Part model, mm, in its own coordinate system. A direction names the side the tool comes from. Give positions to 0.01 mm unless a question says otherwise; leave off trailing zeros. Order: outer loops, then holes, each group sorted by start corner. A loop starts at its lowest first (then second) coordinate and runs counter-clockwise, first axis right, second up. Notation, with made-up numbers: (-7.5, 2) -> (24.5, 2) arc R30 ccw to (24.5, 32) -> close; hole circle Ø1 at (6, 70.25). An arc over 180 degrees is marked (long way). Write item = value, one per line. Start each with the question number.
(1) Saw through at D-D, the plane z = -106. List the corners of the cut face in (x, y), then the cut area to 3 significant figures.
(2) Saw through at A-A, the plane x = -41. State how many separate pieces and enclosed holes the cut face has, then the cut area to 3 significant figures.
(3) Saw through at B-B, the plane y = 33.27. List the corners of the cut face in (x, z), then the cut area to 3 significant figures.
(4) Probe line 1 along Y through (x, z) = (-23.5, -36); line 2 along Z through (x, y) = (-30, 34); line 3 along Y through (x, z) = (-6, -244.5). List the from-to ranges inside material, lowest first. Write a range as from..to.
(5) Flat gauge pins, fed straight in: pin 1 (16 mm diameter, centred on y = -4, z = -25, fed in from -X); pin 2 (1.5 mm diameter, centred on x = 36, z = 215.5, fed in from -Y); pin 3 (8 mm diameter, centred on x = -26.5, y = -24, fed in from +Z). Where does each tip first touch, or does it go through?
(6) Saw through at C-C, the plane z = 37.5. List the corners of the cut face in (x, y).
(7) Two-plate mould, pull along Z, no slides. Class faces 3 (the cylindrical face through (0.833, 31.879, 338.384)), 4 (the cylindrical face through (0.833, -14.175, -62.474)), 5 (the flat face through (-59.5, 7.6, 362.8)): pulls with the +Z half, pulls with the -Z half, needs draft (parallel to the pull), parting line crosses it, or undercut.
(8) Which spindle directions (+Z, -Z, +X, -X, +Y, -Y) get a long thin tool onto all of the face, cutting with end or side? Do faces 1 (the flat face through (-59.5, -39, 97)), 2 (the flat face through (59.5, -13, 174)). Say none if no direction does.
Autodesk Inventor part; units mm, degrees
ref_plane "YZ Plane" through (0, 0, 0) normal (1, 0, 0) x (0, 1, 0)
ref_plane "XZ Plane" through (0, 0, 0) normal (0, 1, 0) x (-1, 0, 0)
ref_plane "XY Plane" through (0, 0, 0) normal (0, 0, 1) x (1, 0, 0)
sketch "Sketch1" plane through (0, 0, 0) normal (1, 0, 0) x (0, 1, 0)
  line L0 (66.79, 404) -> (66.79, -404)
  line L1 (66.79, -404) -> (12.72, -404)
  line L2 (12.72, -404) -> (-46.497, -331.3)
  line L3 (-46.497, -331.3) -> (-46.497, 331.3)
  line L4 (-46.497, 331.3) -> (12.72, 404)
  line L5 (12.72, 404) -> (66.79, 404)
  point P0 (0, 0)
  dimension "d0" = 331.3
  dimension "d1" = 331.3
  dimension "d2" = 46.497
  dimension "d3" = 46.497
  dimension "d4" = 12.72
  dimension "d5" = 12.72
  dimension "d6" = 404
  dimension "d7" = 404
  dimension "d8" = 66.79
extrude "Extrusion1" add sketch "Sketch1" along normal blind 66.5
sketch "Sketch2" plane through (0, 0, 0) normal (-1, 0, 0) x (0, 0, 1)
  line L0 (404, 66.79) -> (-404, 66.79)
  line L1 (-404, 66.79) -> (-404, 12.72)
  line L2 (-404, 12.72) -> (-331.3, -46.497)
  line L3 (331.3, -46.497) -> (404, 12.72)
  line L4 (404, 12.72) -> (404, 66.79)
  line L5 (404, 66.79) -> (-404, 66.79)
  line L6 (-404, 66.79) -> (-404, 12.72)
  line L7 (-404, 12.72) -> (-331.3, -46.497)
  line L8 (-331.3, -46.497) -> (331.3, -46.497)
  point P0 (0, 0)
extrude "Extrusion2" cut sketch "Sketch2" against normal blind 59.5
sketch "Sketch3" plane through (59.5, 0, 0) normal (-1, 0, 0) x (0, 0, 1)
  circle A0 centre (-370.6, 33.27) radius 31.6465
  circle A1 centre (-316, -13.01) radius 31.6465
  circle A2 centre (-246, -13.01) radius 31.6465
  circle A3 centre (-176, -13.01) radius 31.6465
  circle A4 centre (-106, -13.01) radius 31.6465
  circle A5 centre (-36, -13.01) radius 31.6465
  circle A6 centre (34, -13.01) radius 31.6465
  circle A7 centre (104, -13.01) radius 31.6465
  circle A8 centre (174, -13.01) radius 31.6465
  circle A9 centre (244, -13.01) radius 31.6465
  circle A10 centre (314, -13.01) radius 31.6465
  circle A11 centre (370, 33.27) radius 31.6465
  point P0 (0, 0)
  dimension "d13" = 33.27
  dimension "d14" = 33.27
  dimension "d15" = 370.6
  dimension "d16" = 370
  dimension "d17" = 316
  dimension "d18" = 13.01
  dimension "d19" = 70
  dimension "d20" = 70
  dimension "d21" = 70
  dimension "d22" = 70
  dimension "d23" = 70
  dimension "d24" = 70
  dimension "d25" = 70
  dimension "d26" = 70
  dimension "d27" = 70
  dimension "d28" = 13.01
  dimension "d29" = 13.01
  dimension "d30" = 13.01
  dimension "d31" = 13.01
  dimension "d32" = 13.01
  dimension "d33" = 13.01
  dimension "d34" = 13.01
  dimension "d35" = 13.01
  dimension "d36" = 13.01
  dimension "d37" = 63.293
  dimension "d38" = 63.293
  dimension "d39" = 63.293
  dimension "d40" = 63.293
  dimension "d41" = 63.293
  dimension "d42" = 63.293
  dimension "d43" = 63.293
  dimension "d44" = 63.293
  dimension "d45" = 63.293
  dimension "d46" = 63.293
  dimension "d47" = 63.293
  dimension "d48" = 63.293
extrude "Extrusion3" add sketch "Sketch3" along normal blind 119
sketch "Sketch4" plane through (-59.5, 33.27, -370.6) normal (-1, 0, 0) x (0, 0, 1)
  circle A0 centre (0, 0) radius 31.6465
  point P0 (370.6, -33.27)
hole "Hole1" at (-59.5, 33.27, -370.6) direction (1, 0, 0) diameter 53 depth 119
pattern_sketch "Sketch Driven Pattern1" of "Hole1" from (59.5, 33.27, -370.6) copies at (59.5, 33.27, 370) at (59.5, -13.01, -316) at (59.5, -13.01, -246) at (59.5, -13.01, -176) at (59.5, -13.01, -106) at (59.5, -13.01, -36) at (59.5, -13.01, 34) at (59.5, -13.01, 104) at (59.5, -13.01, 174) at (59.5, -13.01, 244) at (59.5, -13.01, 314)
properties part number "Enemy_Track_inertia"
Results list:
q1.outline = (-59.5, -44.66) -> (59.5, -44.66) -> (59.5, -46.5) -> (66.5, -46.5) -> (66.5, 66.79) -> (59.5, 66.79) -> (59.5, 18.64) -> (-59.5, 18.64) -> (-59.5, 13.49) -> (59.5, 13.49) -> (59.5, -39.51) -> (-59.5, -39.51) -> close
q1.area = 2,020 mm^2
q2.separate_pieces = 12
q2.enclosed_holes = 12
q2.area = 11,300 mm^2
q3.outline = (-59.5, -402.25) -> (59.5, -402.25) -> (59.5, -404) -> (66.5, -404) -> (66.5, 404) -> (59.5, 404) -> (59.5, 401.65) -> (-59.5, 401.65) -> (-59.5, 396.5) -> (59.5, 396.5) -> (59.5, 343.5) -> (-59.5, 343.5) -> (-59.5, 338.35) -> (59.5, 338.35) -> (59.5, -338.95) -> (-59.5, -338.95) -> (-59.5, -344.1) -> (59.5, -344.1) -> (59.5, -397.1) -> (-59.5, -397.1) -> close
q3.area = 8,110 mm^2
q4.line_1 = -44.66..-39.51, 13.49..18.64
q4.line_2 = -402.24..-397.09, -344.11..-338.96, 338.36..343.51, 396.49..401.64
q4.line_3 = -44.62..-39.47, 13.45..18.6
q5.pin_1 = 59.5
q5.pin_2 = -28.22
q5.pin_3 = 344.86
q6.outline = (-59.5, -44.46) -> (59.5, -44.46) -> (59.5, -46.5) -> (66.5, -46.5) -> (66.5, 66.79) -> (59.5, 66.79) -> (59.5, 18.44) -> (-59.5, 18.44) -> (-59.5, 13.26) -> (59.5, 13.26) -> (59.5, -39.28) -> (-59.5, -39.28) -> close
q7.face_3 = undercut
q7.face_4 = undercut
q7.face_5 = needs draft
q8.face_1 = +Z, -Z, -X, +Y, -Y
q8.face_2 = -X
